Autodesk Fusion 360 part; units mm, degrees
sketch "Sketch1" plane through (0, 0, 0) normal (0, 1, 0) x (1, 0, 0)
  line L0 (0, 0) -> (65, 0)
  line L1 (65, 0) -> (65, 35)
  line L2 (65, 35) -> (0, 35)
  line L3 (0, 35) -> (0, 0)
  line L4 (10, 35) -> (10, 25) construction
  circle A0 centre (10, 25) radius 7
  dimension "d1" = 35
  dimension "d2" = 65
  dimension "d3" = 14
extrude "Extrude1" add sketch "Sketch1" along normal blind 8
sketch "Sketch2" plane through (0, 8, 0) normal (0, 1, 0) x (-1, 0, 0)
  circle A0 centre (-10, -25) radius 7
  line L0 (0, -35) -> (0, 0)
  line L1 (0, 0) -> (-65, 0)
  line L2 (-65, 0) -> (-65, -35)
  line L3 (-65, -35) -> (0, -35)
  circle A1 centre (-55, -10) radius 5
  dimension "d6" = 10
extrude "Extrude2" cut sketch "Sketch2" against normal blind 4 contours A1
sketch "Sketch3" plane through (0, 0, 0) normal (0, 0, 1) x (1, 0, 0)
  line L0 (0, 0) -> (65, 0)
  line L1 (65, 0) -> (65, 8)
  line L2 (65, 8) -> (0, 8)
  line L3 (0, 8) -> (0, 0)
  line L4 (32.5, 8) -> (35.5, 8)
  line L5 (35.5, 8) -> (35.5, 4)
  line L6 (35.5, 4) -> (29.5, 4)
  line L7 (29.5, 4) -> (29.4914, 8)
  line L8 (32.5, 8) -> (29.4914, 8)
  dimension "d9" = 3
  dimension "d10" = 4
  dimension "d11" = 6
extrude "Extrude3" cut sketch "Sketch3" against normal blind 35 contours L2 L4 L5 L6 L7 L8
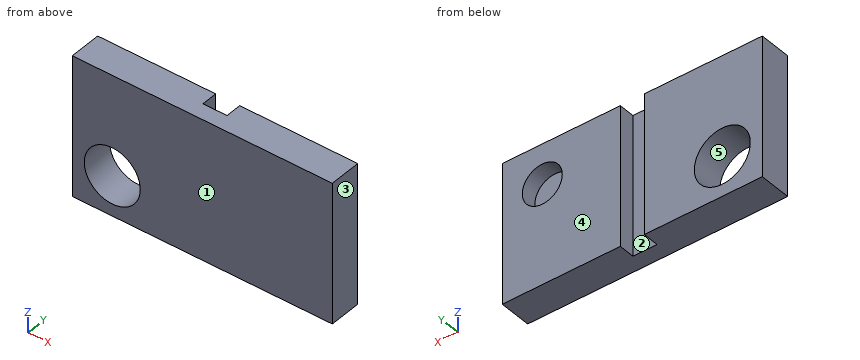
For this review, take the finished solid that the model builds, in its own axes (mm). Face numbers are marked on the shaded views. A direction names the side the tool comes from. Round coordinates to 2 decimals unless told otherwise and drop trailing zeros. Write each loop counter-clockwise with the first axis right and the second up, starting at its lowest first coordinate (ties: lowest second). Pieces come first, ordered by that corner, then holes. Notation, with made-up numbers: M 86.5,-37.5 L 145.5,-37.5 A19 cw 145.5,-33.5 Z; hole C -18.5,6.5 d5. An arc over 180 degrees is marked long. One line per item, written item: value. Start each with the question number.
(1) The part is to be moulded in two halves that separate along X. For the marked faces 3, 4 and 5, say which applies: released by +X, released by -X, zero draft, split by the parting line, or undercut.
(2) Insertion check: pin 1 (3 mm diameter, centred on x = 33, z = -18.5, fed in from +Y); pin 2 (12.5 mm diameter, centred on x = 10, z = -25, fed in from -Y). Each pin has a flat end and moves straight along its axis. Give the tip position at first contact, or say it passes through.
(3) Machinability: for the marked faces 1 and 2, which of the approach directions +Z, -Z, +X, -X, +Y, -Y give a long, thin tool a straight path to every point of the face, cutting with its end or side? Answer none if there is none.
(4) We need section B-B (z = -25). Give the boundary of the cut face in (x, y), and give its area (3 significant figures).
(5) We need section D-D (y = 6.5). Give the boundary of the cut face in (x, z), and give its area (3 significant figures).
(6) Wall thickness on line 1 (X direction, y = 5.75, z = -25); line 2 (Z direction, x = 10, y = 5.5); line 3 (X direction, y = 3.75, z = -25): over which ranges is each line inside the solid? List them lowest first.
(7) We need section C-C (z = -10). Give the boundary of the cut face in (x, y).
(8) We need section A-A (x = 10). Give the boundary of the cut face in (y, z), and give its area (3 significant figures).
Result:
1. face 3: released by +X
1. face 4: zero draft
1. face 5: undercut
2. pin 1: y = 4
2. pin 2: through
3. face 1: +Z, -Z, +X, -X, -Y
3. face 2: +Z, -Z, +Y
4. outline: M 0,0 L 3,0 L 3,8 L 0,8 Z; M 17,0 L 65,0 L 65,8 L 35.5,8 L 35.5,4 L 29.5,4 L 29.49,8 L 17,8 Z
4. area: 384 mm²
5. outline: M 0,-35 L 29.49,-35 L 29.49,0 L 0,0 Z; M 35.5,-35 L 65,-35 L 65,0 L 35.5,0 Z; hole C 10,-25 d14; hole C 55,-10 d10
5. area: 1,830 mm²
6. line 1: 0 to 3, 17 to 29.5, 35.5 to 65
6. line 2: -35 to -32, -18 to 0
6. line 3: 0 to 3, 17 to 65
7. outline: M 0,0 L 65,0 L 65,8 L 60,8 L 60,4 L 50,4 L 50,8 L 35.5,8 L 35.5,4 L 29.5,4 L 29.49,8 L 0,8 Z
8. outline: M 0,-35 L 8,-35 L 8,-32 L 0,-32 Z; M 0,-18 L 8,-18 L 8,0 L 0,0 Z
8. area: 168 mm²
